```python
from build123d import *

# Parameters (mm, degrees)
F0_R      = 9.525
F1_DEPTH  = 38.1
F2_W      = 19.05
F2_H      = 19.05
F3_DEPTH  = 12.7
F4_W      = 19.05
F4_H      = 12.7
F5_DEPTH  = 127
F6_W      = 19.05
F6_H      = 19.05
F7_DEPTH  = 12.7
F8_W      = 19.05
F8_H      = 12.7
F9_DEPTH  = 127
F10_R     = 6.35
F11_DEPTH = 76.2
F12_R     = 6.35
F13_DEPTH = 76.2


with BuildPart() as f1:
    # F0 (on Top) → F1 (new body, symmetric)
    with BuildSketch(Plane.XY):
        Circle(F0_R)
    extrude(amount=F1_DEPTH, both=True)

    # F2 (on face) → F3 (join)
    with BuildSketch(Plane.XY.offset(38.1)):
        Rectangle(F2_W, F2_H)
    extrude(amount=F3_DEPTH)

    # F4 (on face) → F5 (join)
    with BuildSketch(Plane.XZ.offset(9.525)):
        with Locations((0, 44.45)):
            Rectangle(F4_W, F4_H)
    extrude(amount=F5_DEPTH)

    # F6 (on face) → F7 (join)
    with BuildSketch(Plane(origin=(0, 0, -38.1), x_dir=(1, 0, 0), z_dir=(0, 0, -1))):
        Rectangle(F6_W, F6_H)
    extrude(amount=F7_DEPTH)

    # F8 (on face) → F9 (join)
    with BuildSketch(Plane(origin=(0, 9.525, 0), x_dir=(-1, 0, 0), z_dir=(0, 1, 0))):
        with Locations((0, -44.45)):
            Rectangle(F8_W, F8_H)
    extrude(amount=F9_DEPTH)

    # F10 (on face) → F11 (join)
    with BuildSketch(Plane.XY.offset(50.8)):
        with Locations((0, -123.825)):
            Circle(F10_R)
    extrude(amount=F11_DEPTH)

    # F12 (on face) → F13 (join)
    with BuildSketch(Plane(origin=(0, 0, -50.8), x_dir=(1, 0, 0), z_dir=(0, 0, -1))):
        with Locations((0, -123.825)):
            Circle(F12_R)
    extrude(amount=F13_DEPTH)


solid = f1.part
```
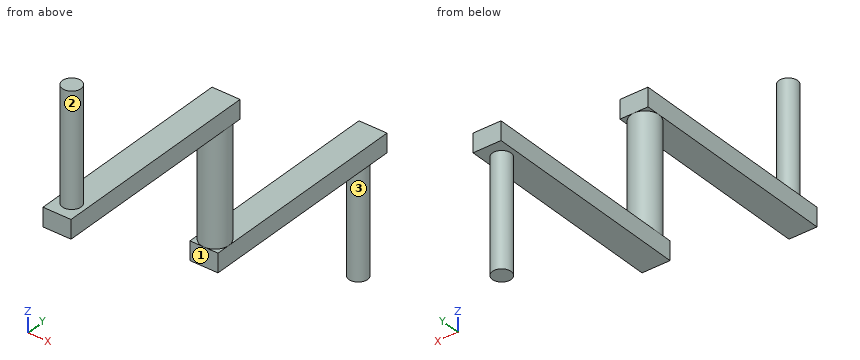
Work out the finished part from the listing and answer in its coordinate system (mm). Face numbers are marked on the shaded views. A direction names the side the tool comes from. Coordinates: 2 decimals unless noted, no trailing zeros. Write each loop counter-clockwise with the first axis right and the second up, starting at its lowest first coordinate (ties: lowest second). Pieces come first, ordered by that corner, then holes.
Q1. A cutting plane is placed at A-A, the plane z = 7.5. Give the vertices of the cut face in (x, y) (3 decimals), then the cut area to 3 significant figures.
Q2. Each of these flat-tipped pins is pushed along its axis until it touches: pin 1 Ø3 at (x, y) = (6, -4) entering from +Z; pin 2 Ø5 at (x, y) = (6.5, 3.5) entering from -Z; pin 3 Ø3 at (x, z) = (-7, -40.5) entering from -Y (3 decimals). Where does it stop, or does it pass through?
Q3. Which of the six approach directions +Z, -Z, +X, -X, +Y, -Y give full straight-line access (tool end or side, diameter ignored) to the marked faces 1, 2 and 3?
Q4. A cutting plane is placed at C-C, the plane z = -94.5. Give the vertices of the cut face in (x, y) (3 decimals), then the cut area to 3 significant figures.
Q5. Find the intervals of material crossed by line 1 (Z direction, x = 7.5, y = -83.5); line 2 (Z direction, x = -6, y = 20); line 3 (Y direction, x = 0.25, z = -84), in increasing order.
Q6. A cutting plane is placed at B-B, the plane y = -22.5. Give the vertices of the cut face in (x, z) (3 decimals).
Findings below:
1. outline: circle Ø19.05 at (0, 0)
1. area: 285 mm2
2. pin 1: stops at z = 50.8
2. pin 2: stops at z = -50.8
2. pin 3: stops at y = -9.525
3. face 1: -Z, +X, -X, -Y
3. face 2: +Z
3. face 3: -Z
4. outline: circle Ø12.7 at (0, 123.825)
4. area: 127 mm2
5. line 1: z = 38.1 to 50.8
5. line 2: z = -50.8 to -38.1
5. line 3: y = 117.48 to 130.17
6. outline: (-9.525, 38.1) - (9.525, 38.1) - (9.525, 50.8) - (-9.525, 50.8) - close
